Input: dimensioned drawing with shaded views. Units: mm. Origin: part minimum x, y, z. A direction names the side the tool comes from. Round coordinates to 2 decimals unless told otherwise and drop trailing zeros. Write each loop counter-clockwise with the first axis right and the second up, starting at its lowest first coordinate (ties: lowest second). Pieces come first, ordered by that corner, then holes. Notation, with made-up numbers: M -10,44 L 41,44 A23 ccw 41,54 Z; hole C 48.25,11 d7. An arc over 180 degrees is marked long. Answer as CSV lines item,"result". Start each with the question number.
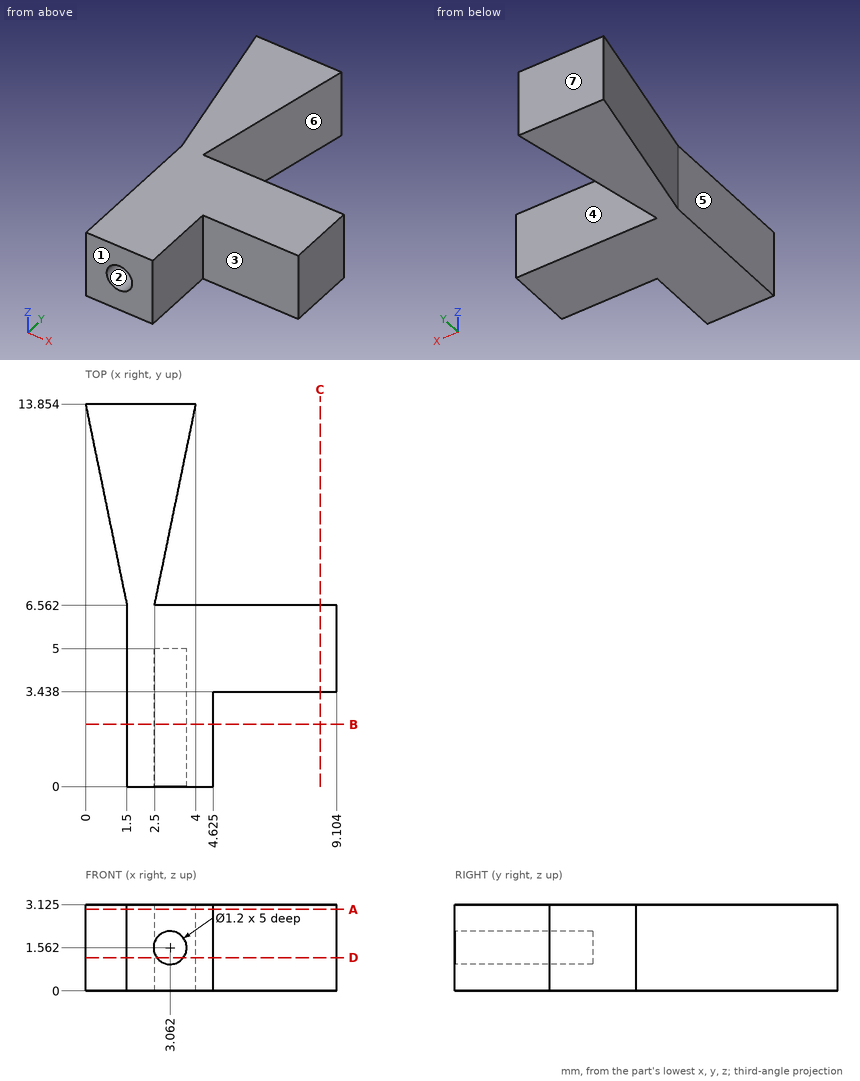
Item 1: Access query for the marked faces 1, 2 and 3. Directions: +Z, -Z, +X, -X, +Y, -Y. A direction counts if a zero-diameter tool reaches every point of the face in a straight line with its end or side. Return the directions, or none.
Item 2: Cut plane D-D, the plane z = 1.2. Return loops of the section in (x, y) (1 decimal).
Item 3: Line query: line 1 (Y direction, x = 6, z = 1.35); line 2 (X direction, y = 6.25, z = 0.9) (1 decimal); line 3 (Y direction, x = 4.25, z = 3.05). Output: solid intervals per line, ascending. Write a range as [from, to].
Item 4: Cut plane B-B, the plane y = 2.25. Return loops of the section in (x, z) (1 decimal).
Item 5: Cut plane C-C, the plane x = 8.5. Return loops of the section in (y, z) (1 decimal).
Item 6: Pin query (flat end, axial travel): pin 1 Ø0.9 at (x, z) = (5, 2) entering from +Y; pin 2 Ø1.5 at (y, z) = (12, 1) entering from +X; pin 3 Ø0.9 at (x, z) = (6.5, 1.5) entering from -Y. Return the tip coordinate at first contact, or that it passes through.
Item 7: Draft query along Y for the marked faces 4, 5, 6 and 7. Return one class per face: +Y half, -Y half, draft (parallel to the pull), parting line (faces both ways), or undercut.
Item 8: Cut plane A-A, the plane z = 2.95. Return loops of the section in (x, y) (1 decimal).
Results list:
1,face 1,"+Z, -Z, +X, -X, -Y"
1,face 2,"-Y"
1,face 3,"+Z, -Z, +X, -Y"
2,outline,"M 0,13.9 L 1.5,6.6 L 1.5,0 L 2.6,0 L 2.6,5 L 3.5,5 L 3.5,0 L 4.6,0 L 4.6,3.4 L 9.1,3.4 L 9.1,6.6 L 2.5,6.6 L 4,13.9 Z"
3,line 1,"[3.44, 6.56]"
3,line 2,"[1.5, 9.1]"
3,line 3,"[0, 6.56]"
4,outline,"M 1.5,0 L 4.6,0 L 4.6,3.1 L 1.5,3.1 Z; hole C 3.1,1.6 d1.2"
5,outline,"M 3.4,0 L 6.6,0 L 6.6,3.1 L 3.4,3.1 Z"
6,pin 1,"y = 6.56"
6,pin 2,"x = 3.77"
6,pin 3,"y = 3.44"
7,face 4,"undercut"
7,face 5,"draft"
7,face 6,"undercut"
7,face 7,"+Y half"
8,outline,"M 0,13.9 L 1.5,6.6 L 1.5,0 L 4.6,0 L 4.6,3.4 L 9.1,3.4 L 9.1,6.6 L 2.5,6.6 L 4,13.9 Z"
